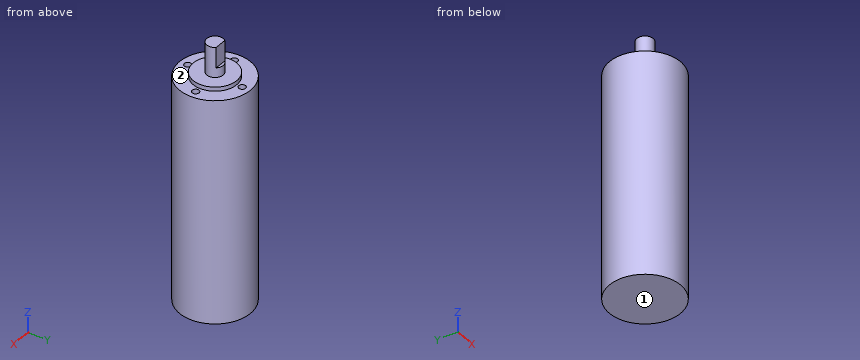
from build123d import *

# Parameters (mm, degrees)
SKETCH1_R           = 26
BOSS_EXTRUDE1_DEPTH = 163.5
SKETCH2_R           = 16
BOSS_EXTRUDE2_DEPTH = 3
SKETCH3_R           = 6
BOSS_EXTRUDE3_DEPTH = 22
CUT_EXTRUDE1_DEPTH  = 15
SKETCH6_R           = 2.5
CUT_EXTRUDE2_DEPTH  = 10


with BuildPart() as part:
    # Sketch1 → Boss-Extrude1 (new body)
    with BuildSketch(Plane.XY):
        Circle(SKETCH1_R)
    extrude(amount=BOSS_EXTRUDE1_DEPTH)

    # Sketch2 → Boss-Extrude2 (add)
    with BuildSketch(Plane.XY.offset(163.5)):
        Circle(SKETCH2_R)
    extrude(amount=BOSS_EXTRUDE2_DEPTH)

    # Sketch3 → Boss-Extrude3 (add)
    with BuildSketch(Plane.XY.offset(166.5)):
        Circle(SKETCH3_R)
    extrude(amount=BOSS_EXTRUDE3_DEPTH)

    # Sketch4 → Cut-Extrude1 (cut)
    with BuildSketch(Plane.XY.offset(188.5)):
        with BuildLine():
            ThreePointArc((0, 6), (-2.449489743, 5.477225575), (-4.472135955, 4))
            Line((-4.472135955, 4), (0, 4))
            Line((0, 4), (0, 6))
        make_face()
        with BuildLine():
            Line((0, 6), (0, 4))
            Line((0, 4), (4.472135955, 4))
            ThreePointArc((4.472135955, 4), (2.449489743, 5.477225575), (0, 6))
        make_face()
    extrude(amount=-CUT_EXTRUDE1_DEPTH, mode=Mode.SUBTRACT)

    # Sketch6 → Cut-Extrude2 (cut)
    with BuildSketch(Plane.XY.offset(163.5)):
        with Locations((0, 20)):
            Circle(SKETCH6_R)
        with Locations((20, 0)):
            Circle(SKETCH6_R)
        with Locations((0, -20)):
            Circle(SKETCH6_R)
        with Locations((-20, 0)):
            Circle(SKETCH6_R)
    extrude(amount=-CUT_EXTRUDE2_DEPTH, mode=Mode.SUBTRACT)


solid = part.part
Work out the finished part from the listing and answer in its coordinate system (mm). Face numbers are marked on the shaded views. A direction names the side the tool comes from. Give positions to 0.01 mm unless a question says otherwise; leave off trailing zeros. Write each loop counter-clockwise with the first axis right and the second up, starting at its lowest first coordinate (ties: lowest second). Pieces come first, ordered by that corner, then holes. Notation, with made-up numbers: M -16.5,22.25 L -10.5,22.25 A23 ccw -10.5,57.25 Z; hole C -2,73 d11. An arc over 180 degrees is marked long. Answer as CSV lines item,"result".
Q1. A cutting plane is placed at D-D on z = 126. Write down the section's boundary in (x, y).
A:
outline,"C 0,0 d52"
Q2. A cutting plane is placed at A-A on x = 0. Write down the section's boundary in (y, z).
A:
outline,"M -26,0 L 26,0 L 26,163.5 L 22.5,163.5 L 22.5,153.5 L 17.5,153.5 L 17.5,163.5 L 16,163.5 L 16,166.5 L 6,166.5 L 6,173.5 L 4,173.5 L 4,188.5 L -6,188.5 L -6,166.5 L -16,166.5 L -16,163.5 L -17.5,163.5 L -17.5,153.5 L -22.5,153.5 L -22.5,163.5 L -26,163.5 Z"
Q3. Find the intervals of material crossed by probe 1 along Y at (x, z) = (0, 159.5); probe 2 along Y at (x, z) = (-0.5, 23); probe 3 along Y at (x, z) = (20, 159), in increasing order. Write a range as [from, to].
A:
probe 1,"y = [-26, -22.5], [-17.5, 17.5], [22.5, 26]"
probe 2,"y = [-26, 26]"
probe 3,"y = [-16.61, -2.5], [2.5, 16.61]"
Q4. A cutting plane is placed at C-C on y = -9.5. Write down the section's boundary in (x, z).
A:
outline,"M -24.2,0 L 24.2,0 L 24.2,163.5 L 12.87,163.5 L 12.87,166.5 L -12.87,166.5 L -12.87,163.5 L -24.2,163.5 Z"
Q5. Given P1, Ø5, axis at y = 7, z = 95, coming from the -X side; P2, Ø1.5, axis at x = 0.5, y = -19.5, coming from the +Z side; P3, Ø3, axis at x = 0, y = -20, coming from the -Z side; P4, Ø6, axis at x = 20, y = 0, coming from the +Z side, each flat-ended and moving along its own axis, determine where each tip first touches the part or whether it passes through.
A:
P1,"stops at x = -25.61"
P2,"stops at z = 153.5"
P3,"stops at z = 0"
P4,"stops at z = 163.5"
Q6. A cutting plane is placed at B-B on z = 159.5. Write down the section's boundary in (x, y).
A:
outline,"C 0,0 d52; hole C -20,0 d5; hole C 0,-20 d5; hole C 0,20 d5; hole C 20,0 d5"
Q7. A tool of negligible diameter and unlimited length cuts with its end or side. For the marked faces 1 and 2, from which of +Z, -Z, +X, -X, +Y, -Y can it reach the whole face along a straight path? Write none if from no direction.
A:
face 1,"-Z, +X, -X, +Y, -Y"
face 2,"+Z"
